Geometry check sheet. Reference: the model listing, model coordinates, mm. Face numbers are marked on the shaded views. A direction names the side the tool comes from. Give positions to 0.01 mm unless a question says otherwise; leave off trailing zeros. Loops run counter-clockwise (first coordinate to the right, second up) from the corner with the lowest first, then second, coordinate; pieces in that order, holes last.
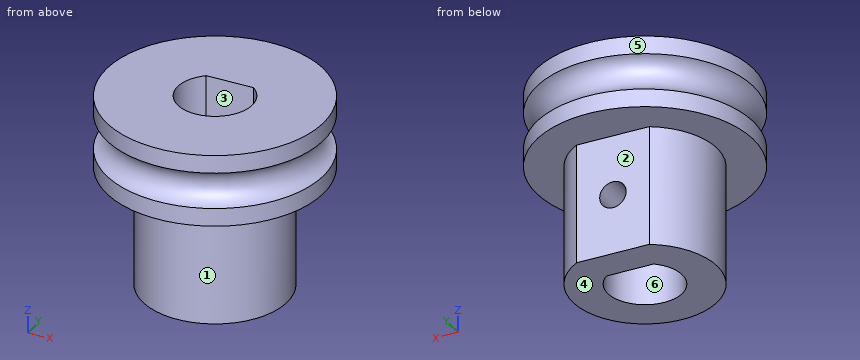
```python
from build123d import *

# Parameters (mm, degrees)
F4_DEPTH = 10
F5_DEPTH = 16.001
F7_D     = 2.2
F7_DEPTH = 4


with BuildPart() as f1:
    # F0 (on Front) → F1 (revolve)
    with BuildSketch(Plane.XZ):
        with BuildLine():
            Line((-9, 0), (0, 0))
            Line((0, 0), (0, 6))
            Line((0, 6), (-9, 6))
            Line((-9, 6), (-9, 4.5))
            ThreePointArc((-9, 4.5), (-7.8, 3), (-9, 1.5))
            Line((-9, 1.5), (-9, 0))
        make_face()
    revolve(axis=Axis((0, 0, 3), (0, 0, 1)))

    # F3 (on Top) → F4 (join)
    with BuildSketch(Plane.XY):
        with BuildLine():
            Line((3.0351, 5.175729), (-3.0351, 5.175729))
            ThreePointArc((-3.0351, 5.175729), (0, -6), (3.0351, 5.175729))
        make_face()
    extrude(amount=-F4_DEPTH)

    # F2 (on face) → F5 (cut, through all)
    with BuildSketch(Plane.XY.offset(6)):
        with BuildLine():
            Line((1.967733, 2.395418), (-1.967733, 2.395418))
            ThreePointArc((-1.967733, 2.395418), (0, -3.1), (1.967733, 2.395418))
        make_face()
    extrude(amount=-F5_DEPTH, mode=Mode.SUBTRACT)

    # F7
    with Locations(Plane(origin=(0, 5.175729, 0), x_dir=(-1, 0, 0), z_dir=(0, 1, 0))):
        with Locations((0, -5)):
            Hole(F7_D / 2, depth=F7_DEPTH)


solid = f1.part
```
1) Sectioned sample at B-B on y = 0. Enter the section's corners in (x, z) (1 decimal), plus the area to 3 significant figures.
2) Sectioned sample at A-A on x = 0. Enter the section's corners in (y, z) (1 decimal), plus the area to 3 significant figures.
3) Depth check by flat-ended pin: P1, Ø1.2, axis at x = -0.5, z = -5, coming from the -Y side; P2, Ø1, axis at x = 5.5, z = -4.5, coming from the +Y side; P3, Ø1, axis at x = 5.5, z = 0.5, coming from the +Y side. Enter the tip coordinate at first touch or a pass-through.
4) Scan lines: line 1 along Z through (x, y) = (0, 3.85); line 2 along X through (y, z) = (-2.25, -1.75); line 3 along X through (y, z) = (0, 2.75). Record each from-to range of solid material in increasing order.
5) Sectioned sample at D-D on z = -0.5. Enter the section's corners in (x, y), plus the area to 3 significant figures.
6) Sectioned sample at C-C on z = -5. Enter the section's corners in (x, y), plus the area to 3 significant figures.
7) Mould release check, pull along Y, two halves, no side actions. Record for the marked faces 4, 5 and 6: +Y half, -Y half, draft (parallel to the pull), parting line (faces both ways), or undercut.
8) Tool access check on the marked faces 1, 2 and 3. Record the directions out of +Z, -Z, +X, -X, +Y, -Y that give a thin tool (end or side, any length) a straight path to the whole face; none if there is none.
Determined:
1. outline: (-9, 0) - (-6, 0) - (-6, -10) - (-3.1, -10) - (-3.1, 6) - (-9, 6) - (-9, 4.5) arc R1.5 cw to (-9, 1.5) - close; (3.1, -10) - (6, -10) - (6, 0) - (9, 0) - (9, 1.5) arc R1.5 cw to (9, 4.5) - (9, 6) - (3.1, 6) - close
1. area: 123 mm2
2. outline: (-9, 0) - (-6, 0) - (-6, -10) - (-3.1, -10) - (-3.1, 6) - (-9, 6) - (-9, 4.5) arc R1.5 cw to (-9, 1.5) - close; (2.4, -10) - (5.2, -10) - (5.2, -6.1) - (2.4, -6.1) - close; (2.4, -3.9) - (5.2, -3.9) - (5.2, 0) - (9, 0) - (9, 1.5) arc R1.5 cw to (9, 4.5) - (9, 6) - (2.4, 6) - close
2. area: 120 mm2
3. P1: stops at y = -6
3. P2: stops at y = 3.32
3. P3: stops at y = 7.48
4. line 1: z = -10 to -6.1, -3.9 to 6
4. line 2: x = -5.56 to -2.13, 2.13 to 5.56
4. line 3: x = -7.82 to -3.1, 3.1 to 7.82
5. outline: (-3.04, 5.18) arc R6 ccw (long way) to (3.04, 5.18) - close; hole (-1.97, 2.4) arc R3.1 ccw (long way) to (1.97, 2.4) - close
5. area: 81.4 mm2
6. outline: (-3.04, 5.18) arc R6 ccw (long way) to (3.04, 5.18) - (1.1, 5.18) - (1.1, 2.4) - (1.97, 2.4) arc R3.1 cw (long way) to (-1.97, 2.4) - (-1.1, 2.4) - (-1.1, 5.18) - close
6. area: 75.3 mm2
7. face 4: draft
7. face 5: parting line
7. face 6: undercut
8. face 1: -Z
8. face 2: -Z, +X, -X, +Y
8. face 3: +Z, -Z
